Autodesk Inventor part; units mm, degrees
ref_plane "Work Plane1" through (0, 9.525, 0) normal (0, 1, 0) x (-1, 0, 0)
ref_plane "YZ Plane" through (0, 0, 0) normal (1, 0, 0) x (0, 1, 0)
ref_plane "XY Plane" through (0, 0, 0) normal (0, 0, 1) x (1, 0, 0)
sketch "Sketch1" plane through (0, 0, 0) normal (0, 0, 1) x (1, 0, 0)
  line L0 (2.7496, 4.7625) -> (5.4993, 0)
  line L1 (5.4993, 0) -> (2.7496, -4.7625)
  line L2 (2.7496, -4.7625) -> (-2.7496, -4.7625)
  line L3 (-2.7496, -4.7625) -> (-5.4993, 0)
  line L4 (-5.4993, 0) -> (-2.7496, 4.7625)
  line L5 (-2.7496, 4.7625) -> (2.7496, 4.7625)
  circle A0 centre (0, 0) radius 9.525
  circle A1 centre (0, 0) radius 5.4993 construction
  dimension "d0" = 9.525
  dimension "d2" = 19.05
  dimension "d3" = 4.0257
extrude "Extrusion1" add sketch "Sketch1" against normal blind 19.05
thicken "Thicken Hex" operation add thickness 0.127 both sides no extend neighbours yes toward (-0.8660254, 0.5, 0) faces at (-4.5827, 1.5875, -6.35) (-3.6662, -3.175, -6.35) (0.9165, -4.7625, -6.35) (-0.9165, 4.7625, -6.35) (3.6662, 3.175, -6.35) (4.5827, -1.5875, -6.35)
sketch "Sketch3" plane through (0, 0, 0) normal (0, 0, 1) x (1, 0, 0)
  line L0 (5.6459, 0) -> (2.823, -4.8895)
  line L1 (2.823, -4.8895) -> (-2.823, -4.8895)
  line L2 (-2.823, -4.8895) -> (-5.6459, 0)
  line L3 (-5.6459, 0) -> (-2.823, 4.8895)
  line L4 (-2.823, 4.8895) -> (2.823, 4.8895)
  line L5 (2.823, 4.8895) -> (5.6459, 0)
  line L6 (2.823, 4.8895) -> (5.6459, 0)
  circle A0 centre (0, 0) radius 6.35
  dimension "d10" = 12.7
extrude "Extrusion2" add sketch "Sketch3" along normal blind 12.7
thicken "Thicken2" operation add thickness 0.127 both sides no extend neighbours yes toward (-0.9967573, 0.0804666, 0) faces at (6.3294, -0.511, 8.4667)
ref_plane "Work Plane1" through (0, 9.525, 0) normal (0, 1, 0) x (-1, 0, 0)
sketch "Sketch4" plane through (0, 9.525, 0) normal (0, 1, 0) x (-1, 0, 0)
  line L0 (0, 0) -> (0, -19.05) construction
  line L1 (2.823, -19.05) -> (-2.823, -19.05) construction
  point P0 (0, -9.525)
hole "Hole1" at (0, 9.525, -9.525) direction (0, -1, 0) diameter 3.81 end through all
equation "\"d0\" = hexSize"
equation "\"d2\" = exteriorDiameter"
equation "\"d4\" = length"
equation "\"d6\" = printSpacing"
equation "\"d7\" = printSpacing"
equation "\"d10\" = baseBushingDiameter"
equation "\"d8\" = baseBushingLength"
equation "\"d11\" = printSpacing"
equation "\"d12\" = printSpacing"
equation "\"hexSize\" = 9.525"
equation "\"exteriorDiameter\" = 19.05"
equation "\"length\" = 19.05"
equation "\"printSpacing\" = 0.127"
equation "\"baseBushingDiameter\" = 12.7"
equation "\"baseBushingLength\" = 12.7"
properties part number "3_8x3_4x3_4-hexBearingEndCap" material "PC/ABS Plastic"
The model under review builds one solid part; all positions refer to its coordinate system, in mm. A direction names the side the tool comes from. Round coordinates to 2 decimals unless told otherwise and drop trailing zeros. Order: outer loops, then holes, each group sorted by start corner. A loop starts at its lowest first (then second) coordinate and runs counter-clockwise, first axis right, second up. Notation, with made-up numbers: (-13.75, 62) -> (-3.75, 62) arc R17 ccw to (-3.75, 81) -> close; hole circle Ø4 at (-8, 67.25). An arc over 180 degrees is marked (long way). Use a Markdown table: item, result.
Q1. We need section B-B on x = 0. State how many separate pieces and enclosed holes the cut face has, then the cut area to 3 significant figures.
Values:
| item | result |
|---|---|
| separate pieces | 4 |
| enclosed holes | 0 |
| area | 175 mm^2 |
Q2. Mouldability with a two-part tool opening along Z and no side actions: class faces 4 (the cylindrical face through (-0.572, -7.24, -7.708)), 5 (the flat face through (4, -4, -19.05)), 6 (the flat face through (0, 4.89, -3)) as +Z half, -Z half, draft (parallel to the pull), parting line (faces both ways), or undercut.
Values:
| item | result |
|---|---|
| face 4 | undercut |
| face 5 | -Z half |
| face 6 | draft |
Q3. We need section C-C on x = -3.5. Write out the cut boundary in (y, z).
Values:
| item | result |
|---|---|
| outline | (-8.86, -19.05) -> (-3.72, -19.05) -> (-3.72, 12.7) -> (-5.15, 12.7) -> (-5.15, 0) -> (-8.86, 0) -> close; (3.72, -19.05) -> (8.86, -19.05) -> (8.86, 0) -> (5.15, 0) -> (5.15, 12.7) -> (3.72, 12.7) -> close |
Q4. We need section D-D on y = -0.5. Write out the cut boundary in (x, z), then the cut area to 3 significant figures.
Values:
| item | result |
|---|---|
| outline | (-9.51, -19.05) -> (-5.36, -19.05) -> (-5.36, 12.7) -> (-6.2, 12.7) -> (-6.2, 0) -> (-9.51, 0) -> close; (5.36, -19.05) -> (9.51, -19.05) -> (9.51, 0) -> (6.2, 0) -> (6.2, 12.7) -> (5.36, 12.7) -> close |
| area | 180 mm^2 |
Q5. Clearance check with flat-ended pins moving along their axes: P1, Ø2, axis at y = 1.5, z = -12, coming from the -X side; P2, Ø1, axis at x = 5.5, z = 8.5, coming from the -Y side. State where each tip first meets the part, or that it passes through.
Values:
| item | result |
|---|---|
| P1 | stops at x = -9.51 |
| P2 | stops at y = -3.7 |
Q6. For line 1 (Z direction, x = 0, y = 8.1); line 2 (Y direction, x = -5.5, z = 7); line 3 (X direction, y = 2, z = -4), list the stretches that pass through material, from the lowest coordinate up.
Values:
| item | result |
|---|---|
| line 1 | z = -19.05 to -11.43, -7.62 to 0 |
| line 2 | y = -2.91 to -0.25, 0.25 to 2.91 |
| line 3 | x = -9.31 to -4.49, 4.49 to 9.31 |
Q7. Tool access review of faces 1 (the flat face through (-0.5, 5.1, 12.7)), 2 (the flat face through (0, -4.89, -3)), 3 (the flat face through (6.2, -2, 0)): name each direction out of +Z, -Z, +X, -X, +Y, -Y from which nothing blocks a thin tool from reaching the whole face with its end or side.
Values:
| item | result |
|---|---|
| face 1 | +Z, +X, -X, +Y, -Y |
| face 2 | +Z, -Z |
| face 3 | +Z |
